Check sheet for the modelled part. Datum: model origin and axes. Units: mm. Round coordinates to 2 decimals unless told otherwise and drop trailing zeros. Write each loop counter-clockwise with the first axis right and the second up, starting at its lowest first coordinate (ties: lowest second). Pieces come first, ordered by that corner, then holes. Notation, with made-up numbers: (-36.5, 59) -> (11.5, 59) arc R25 ccw to (11.5, 85) -> close; hole circle Ø7 at (-30, -31). An arc over 180 degrees is marked (long way). One line per item, written item: value.
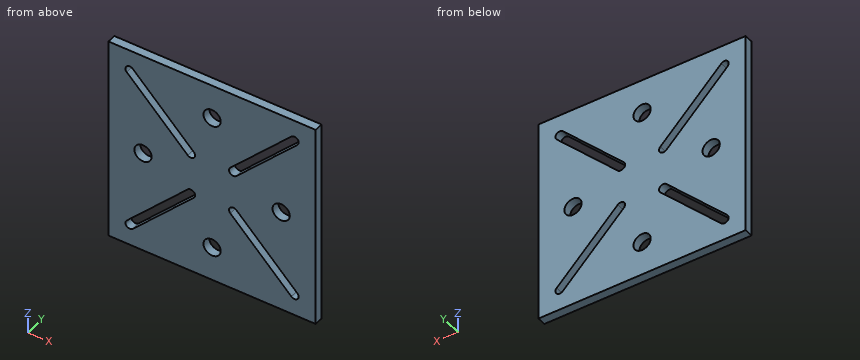
from build123d import *

# Parameters (mm, degrees)
SKETCH1_W           = 152.4
SKETCH1_H           = 152.4
SKETCH1_R           = 6.35
BOSS_EXTRUDE1_DEPTH = 6.35


with BuildPart() as part:
    # Sketch1 → Boss-Extrude1 (new body)
    with BuildSketch(Plane(origin=(0, 0, 0), x_dir=(1, 0, 0), z_dir=(0, 1, 0))):
        with Locations((76.2, 76.2)):
            Rectangle(SKETCH1_W, SKETCH1_H)
        with Locations(Location((25.4, 76.2, 0), (0, 0, 270))):
            Circle(SKETCH1_R, mode=Mode.SUBTRACT)
        with Locations(Location((76.2, 127, 0), (0, 0, 270))):
            Circle(SKETCH1_R, mode=Mode.SUBTRACT)
        with Locations(Location((127, 76.2, 0), (0, 0, 270))):
            Circle(SKETCH1_R, mode=Mode.SUBTRACT)
        with Locations(Location((76.2, 25.4, 0), (0, 0, 270))):
            Circle(SKETCH1_R, mode=Mode.SUBTRACT)
        with BuildLine():
            Line((17.894423728, 138.995704333), (62.795704333, 94.094423728))
            ThreePointArc((62.795704333, 94.094423728), (62.795704333, 89.604295667), (58.305576272, 89.604295667))
            Line((58.305576272, 89.604295667), (13.404295667, 134.505576272))
            ThreePointArc((13.404295667, 134.505576272), (13.404295667, 138.995704333), (17.894423728, 138.995704333))
        make_face(mode=Mode.SUBTRACT)
        with BuildLine():
            Line((134.505576272, 138.995704333), (89.604295667, 94.094423728))
            ThreePointArc((89.604295667, 94.094423728), (89.604295667, 89.604295667), (94.094423728, 89.604295667))
            Line((94.094423728, 89.604295667), (138.995704333, 134.505576272))
            ThreePointArc((138.995704333, 134.505576272), (138.995704333, 138.995704333), (134.505576272, 138.995704333))
        make_face(mode=Mode.SUBTRACT)
        with BuildLine():
            Line((134.505576272, 13.404295667), (89.604295667, 58.305576272))
            ThreePointArc((89.604295667, 58.305576272), (89.604295667, 62.795704333), (94.094423728, 62.795704333))
            Line((94.094423728, 62.795704333), (138.995704333, 17.894423728))
            ThreePointArc((138.995704333, 17.894423728), (138.995704333, 13.404295667), (134.505576272, 13.404295667))
        make_face(mode=Mode.SUBTRACT)
        with BuildLine():
            Line((17.894423728, 13.404295667), (62.795704333, 58.305576272))
            ThreePointArc((62.795704333, 58.305576272), (62.795704333, 62.795704333), (58.305576272, 62.795704333))
            Line((58.305576272, 62.795704333), (13.404295667, 17.894423728))
            ThreePointArc((13.404295667, 17.894423728), (13.404295667, 13.404295667), (17.894423728, 13.404295667))
        make_face(mode=Mode.SUBTRACT)
    extrude(amount=BOSS_EXTRUDE1_DEPTH)


solid = part.part
Item 1: Depth check by flat-ended pin: P1, Ø7.5, axis at x = 76.2, z = -25.4, coming from the -Y side. Enter the tip coordinate at first touch or a pass-through.
Answer:
P1: passes through
Item 2: Sectioned sample at D-D on z = -25.4. Enter the section's corners in (x, y), and give its area (3 significant figures).
Answer:
outline: (0, 0) -> (20.91, 0) -> (20.91, 6.35) -> (0, 6.35) -> close; (29.89, 0) -> (69.85, 0) -> (69.85, 6.35) -> (29.89, 6.35) -> close; (82.55, 0) -> (122.51, 0) -> (122.51, 6.35) -> (82.55, 6.35) -> close; (131.49, 0) -> (152.4, 0) -> (152.4, 6.35) -> (131.49, 6.35) -> close
area: 773 mm^2
Item 3: Thickness scan on line 1 (X direction, y = 2.75, z = -76.2); line 2 (X direction, y = 0.75, z = -42.5); line 3 (X direction, y = 2.75, z = -25.4). Record the ranges inside material, lowest first.
Answer:
line 1: x = 0 to 19.05, 31.75 to 120.65, 133.35 to 152.4
line 2: x = 0 to 38.01, 46.99 to 105.41, 114.39 to 152.4
line 3: x = 0 to 20.91, 29.89 to 69.85, 82.55 to 122.51, 131.49 to 152.4
Item 4: Sectioned sample at B-B on x = 76.2. Enter the section's corners in (y, z).
Answer:
outline: (0, -152.4) -> (6.35, -152.4) -> (6.35, -133.35) -> (0, -133.35) -> close; (0, -120.65) -> (6.35, -120.65) -> (6.35, -31.75) -> (0, -31.75) -> close; (0, -19.05) -> (6.35, -19.05) -> (6.35, 0) -> (0, 0) -> close
Item 5: Sectioned sample at C-C on y = 3. Count the separate pieces of the cut face and the enclosed holes in it, and give its area (3 significant figures).
Answer:
separate pieces: 1
enclosed holes: 8
area: 21,000 mm^2
Item 6: Sectioned sample at A-A on z = -76.2. Enter the section's corners in (x, y).
Answer:
outline: (0, 0) -> (19.05, 0) -> (19.05, 6.35) -> (0, 6.35) -> close; (31.75, 0) -> (120.65, 0) -> (120.65, 6.35) -> (31.75, 6.35) -> close; (133.35, 0) -> (152.4, 0) -> (152.4, 6.35) -> (133.35, 6.35) -> close
